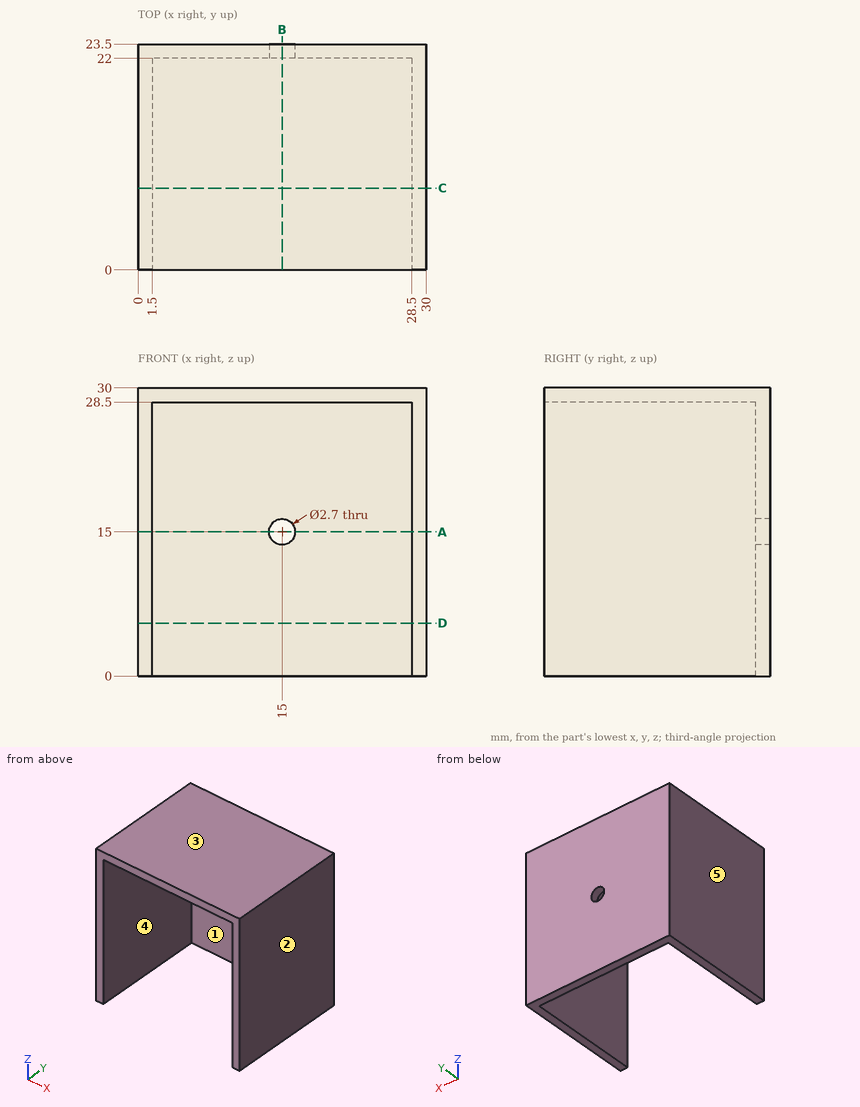
Geometry check sheet. Reference: drawing and pictorial views, mm from the part's lowest x, y, z. A direction names the side the tool comes from. Give positions to 0.01 mm unless a question says otherwise; leave off trailing zeros. Loops run counter-clockwise (first coordinate to the right, second up) from the corner with the lowest first, then second, coordinate; pieces in that order, holes last.
1. Mould release check, pull along X, two halves, no side actions. Record for the marked faces 3, 4 and 5: released by +X, released by -X, zero draft, split by the parting line, or undercut.
2. Section check A-A, the plane z = 15. Enter the section's corners in (x, y), then the cut area to 3 significant figures.
3. Section check C-C, the plane y = 8.5. Enter the section's corners in (x, z), then the cut area to 4 significant figures.
4. Section check B-B, the plane x = 15. Enter the section's corners in (y, z), then the cut area to 4 significant figures.
5. Set-up check for the marked faces 1 and 2: record each of +Z, -Z, +X, -X, +Y, -Y from which the full face is reachable in a straight line by a thin tool's end or side.
6. Section check D-D, the plane z = 5.5. Enter the section's corners in (x, y), then the cut area to 3 significant figures.
7. Go/stop test with a flat-tipped pin: pin 1 Ø1 at (x, z) = (10.5, 9) entering from -Y. Record where the tip stops, or that it passes through.
8. Thickness scan on line 1 (X direction, y = 3, z = 7.5); line 2 (X direction, y = 22.65, z = 15). Record the ranges inside material, lowest first.
Geometry says:
1. face 3: zero draft
1. face 4: undercut
1. face 5: released by -X
2. outline: (0, 0) - (1.5, 0) - (1.5, 22) - (13.65, 22) - (13.65, 23.5) - (0, 23.5) - close; (16.35, 22) - (28.5, 22) - (28.5, 0) - (30, 0) - (30, 23.5) - (16.35, 23.5) - close
2. area: 107 mm2
3. outline: (0, 0) - (1.5, 0) - (1.5, 28.5) - (28.5, 28.5) - (28.5, 0) - (30, 0) - (30, 30) - (0, 30) - close
3. area: 130.5 mm2
4. outline: (0, 28.5) - (22, 28.5) - (22, 16.35) - (23.5, 16.35) - (23.5, 30) - (0, 30) - close; (22, 0) - (23.5, 0) - (23.5, 13.65) - (22, 13.65) - close
4. area: 73.95 mm2
5. face 1: -Z, -Y
5. face 2: +Z, -Z, +X, +Y, -Y
6. outline: (0, 0) - (1.5, 0) - (1.5, 22) - (28.5, 22) - (28.5, 0) - (30, 0) - (30, 23.5) - (0, 23.5) - close
6. area: 111 mm2
7. pin 1: stops at y = 22
8. line 1: x = 0 to 1.5, 28.5 to 30
8. line 2: x = 0 to 13.65, 16.35 to 30
